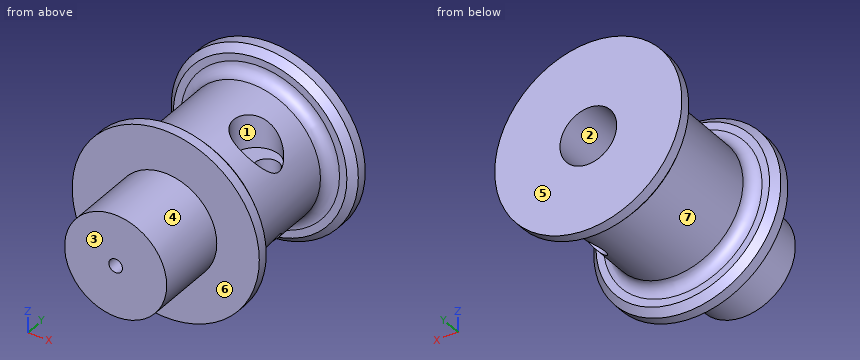
```python
from build123d import *

# Parameters (mm, degrees)
F_10_24_TAPPED_HOLE1_D  = 3.7973
CHAMFER1_SIZE           = 1.905
FILLET1_R               = 3.175
SKETCH5_R               = 7.9375
CUT_EXTRUDE2_DEPTH      = 56.67375
SKETCH6_R               = 3.3782
CUT_EXTRUDE3_DEPTH      = 27.19375
CUT_EXTRUDE3_DEPTH_BACK = 27.19375
CUT_EXTRUDE4_START      = 8.845327
SKETCH7_R               = 6.35
CUT_EXTRUDE4_DEPTH      = 18.348423


with BuildPart() as part:
    # Sketch1 → Revolve1 (revolve)
    with BuildSketch(Plane.XY):
        Polygon((0, 0), (14.2875, 0), (14.2875, 20.6375), (26.19375, 20.6375), (26.19375, 25.4), (19.05, 25.4), (19.05, 59.53125), (26.19375, 59.53125), (26.19375, 64.29375), (0, 64.29375), align=None)
    revolve(axis=Axis((0, 64.29375, 0), (0, -1, 0)))

    # #10-24 Tapped Hole1 (through all)
    with Locations(Plane(origin=(0, 64.29375, 0), x_dir=(1, 0, 0), z_dir=(0, 1, 0))):
        with Locations((0, 0)):
            Hole(F_10_24_TAPPED_HOLE1_D / 2)

    # Chamfer1
    chamfer1_edges = [part.edges().sort_by_distance(p)[0] for p in [
        (-26.19375, 59.53125, 0),
        (-26.19375, 25.4, 0),
    ]]
    chamfer(chamfer1_edges, length=CHAMFER1_SIZE)

    # Fillet1
    fillet1_edges = [part.edges().sort_by_distance(p)[0] for p in [
        (-19.05, 59.53125, 0),
        (-19.05, 25.4, 0),
    ]]
    fillet(fillet1_edges, radius=FILLET1_R)

    # Sketch5 → Cut-Extrude2 (cut)
    with BuildSketch(Plane(origin=(0, 64.29375, 0), x_dir=(1, 0, 0), z_dir=(0, 1, 0))):
        Circle(SKETCH5_R)
    extrude(amount=-CUT_EXTRUDE2_DEPTH, mode=Mode.SUBTRACT)

    # Sketch6 → Cut-Extrude3 (cut, two sides)
    with BuildSketch(Plane.XY) as cut_extrude3_sk:
        with Locations((13.49375, 42.465625)):
            Circle(SKETCH6_R)
    extrude(amount=CUT_EXTRUDE3_DEPTH, mode=Mode.SUBTRACT)
    extrude(cut_extrude3_sk.sketch, amount=-CUT_EXTRUDE3_DEPTH_BACK, mode=Mode.SUBTRACT)

    # Sketch7 → Cut-Extrude4 (cut, through all)
    with BuildSketch(Plane.XY.offset(CUT_EXTRUDE4_START)):
        with Locations((10.52195, 42.465625)):
            Circle(SKETCH7_R)
    extrude(amount=CUT_EXTRUDE4_DEPTH, mode=Mode.SUBTRACT)


solid = part.part
```
Geometry check sheet. Reference: the model listing, model coordinates, mm. Face numbers are marked on the shaded views. A direction names the side the tool comes from. Coordinates: 2 decimals unless noted, no trailing zeros. Order: outer loops, then holes, each group sorted by start corner. A loop starts at its lowest first (then second) coordinate and runs counter-clockwise, first axis right, second up.
Item 1: Section check C-C (z = -1). Count the separate pieces of the cut face and the enclosed holes in it, plus the area to 3 significant figures.
Item 2: Depth check by flat-ended pin: pin 1 (8 mm diameter, centred on x = 11.5, y = 24.5, fed in from +Z); pin 2 (14 mm diameter, centred on x = 11, y = 44.5, fed in from +Z); pin 3 (8 mm diameter, centred on y = 50.5, z = 20.5, fed in from +X). Enter the tip coordinate at first touch or a pass-through.
Item 3: Scan lines: line 1 along X through (y, z) = (42, -1); line 2 along Y through (x, z) = (10.5, 11.5); line 3 along Z through (x, y) = (0, 4.75). Record each from-to range of solid material in increasing order.
Item 4: Mould release check, pull along Y, two halves, no side actions. Record for the marked faces 5, 6 and 7: released by +Y, released by -Y, zero draft, split by the parting line, or undercut.
Item 5: Section check B-B (y = 22). Enter the section's corners in (x, z) (1 decimal), plus the area to 3 significant figures.
Item 6: Tool access check on the marked faces 1, 2, 3 and 4. Record the directions out of +Z, -Z, +X, -X, +Y, -Y that give a thin tool (end or side, any length) a straight path to the whole face; none if there is none.
Check sheet entries:
1. separate pieces: 2
1. enclosed holes: 1
1. area: 1,430 mm2
2. pin 1: stops at z = 25.06
2. pin 2: stops at z = 18.63
2. pin 3: stops at x = 9.52
3. line 1: x = -19.02 to -7.87, 7.87 to 10.15, 16.84 to 19.02
3. line 2: y = 20.64 to 36.12, 48.82 to 64.29
3. line 3: z = -14.29 to -1.9, 1.9 to 14.29
4. face 5: released by +Y
4. face 6: released by -Y
4. face 7: undercut
5. outline: circle Ø52.4 at (0, 0); hole circle Ø15.9 at (0, 0)
5. area: 1,960 mm2
6. face 1: +Z
6. face 2: +Y
6. face 3: +Z, -Z, +X, -X, -Y
6. face 4: -Y
